Drawing for the job (mm, zero at the part's lowest x, y, z). Round coordinates to 2 decimals unless told otherwise and drop trailing zeros. Loops run counter-clockwise (first coordinate to the right, second up) from the corner with the lowest first, then second, coordinate; pieces in that order, holes last.
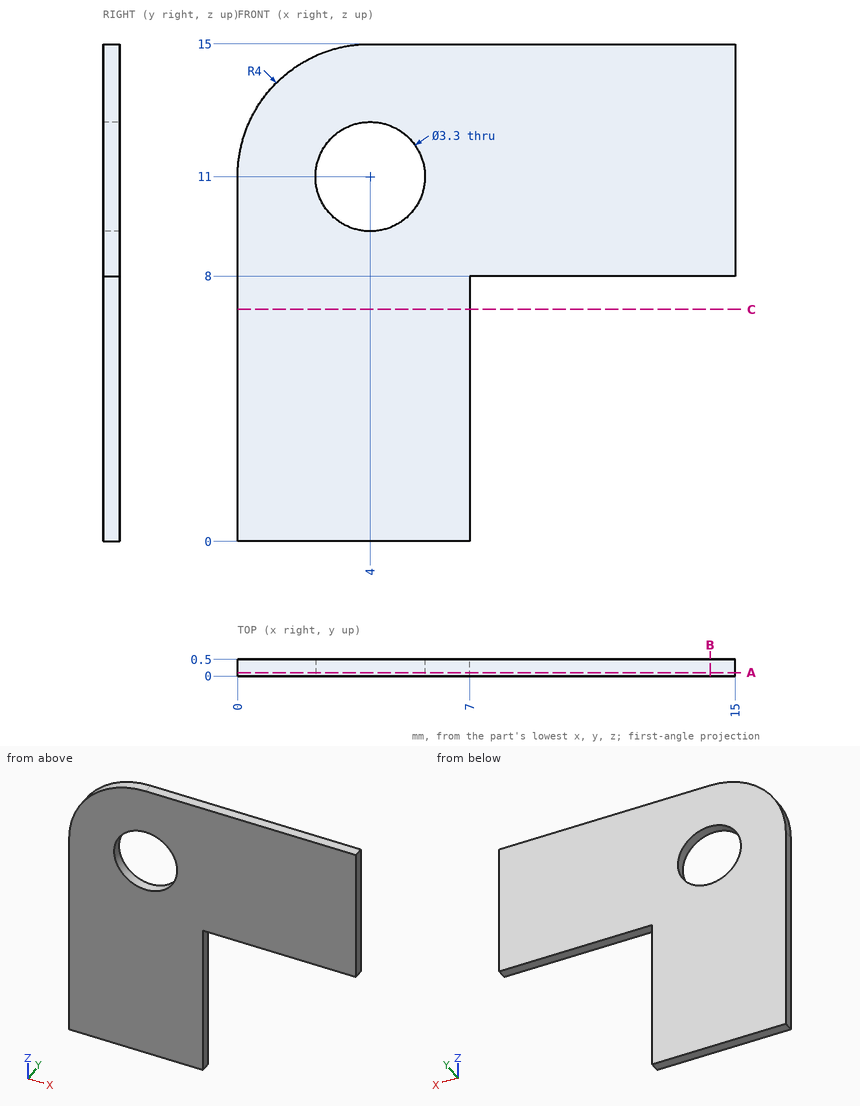
Q1. Slice it at A-A on y = 0.1. Give the cut face in (x, z).
Q2. Probe line 1 (X direction, y = 0.1, z = 11); line 2 (X direction, y = 0.1, z = 4); line 3 (X direction, y = 0.35, z = 11.5). List the from-to ranges inside material, lowest first.
Q3. Slice it at C-C on z = 7. Give the cut face in (x, y).
Q4. Slice it at B-B on x = 14.25. Give the cut face in (y, z).
Reply:
1. outline: (0, 0) - (7, 0) - (7, 8) - (15, 8) - (15, 15) - (4, 15) arc R4 ccw to (0, 11) - close; hole circle Ø3.3 at (4, 11)
2. line 1: x = 0 to 2.35, 5.65 to 15
2. line 2: x = 0 to 7
2. line 3: x = 0.03 to 2.43, 5.57 to 15
3. outline: (0, 0) - (7, 0) - (7, 0.5) - (0, 0.5) - close
4. outline: (0, 8) - (0.5, 8) - (0.5, 15) - (0, 15) - close
